from build123d import *

# Parameters (mm, degrees)
SKETCH1_R           = 3.7
BOSS_EXTRUDE1_DEPTH = 3.9
CUT_EXTRUDE1_DEPTH  = 10.392550239
CHAMFER1_SIZE       = 0.4


with BuildPart() as part:
    # Sketch1 → Boss-Extrude1 (new, symmetric)
    with BuildSketch(Plane(origin=(0, 0, 0), x_dir=(1, 0, 0), z_dir=(0, 1, 0))):
        with Locations(Location((0, 0, 0), (0, 0, 270))):
            Circle(SKETCH1_R)
    extrude(amount=BOSS_EXTRUDE1_DEPTH, both=True)

    # Sketch2 → Cut-Extrude1 (cut, through all)
    with BuildSketch(Plane(origin=(0, 3.9, 0), x_dir=(1, 0, 0), z_dir=(0, 1, 0))):
        Polygon((0.925, 0.925), (2.4, 0.925), (2.4, -0.925), (0.925, -0.925), (0.925, -2.4), (-0.925, -2.4), (-0.925, -0.925), (-2.4, -0.925), (-2.4, 0.925), (-0.925, 0.925), (-0.925, 2.4), (0.925, 2.4), align=None)
    extrude(amount=-CUT_EXTRUDE1_DEPTH, mode=Mode.SUBTRACT)

    # Chamfer1
    chamfer1_edges = [part.edges().sort_by_distance(p)[0] for p in [
        (0, -3.9, -3.7),
        (0, 3.9, -3.7),
    ]]
    chamfer(chamfer1_edges, length=CHAMFER1_SIZE)


solid = part.part
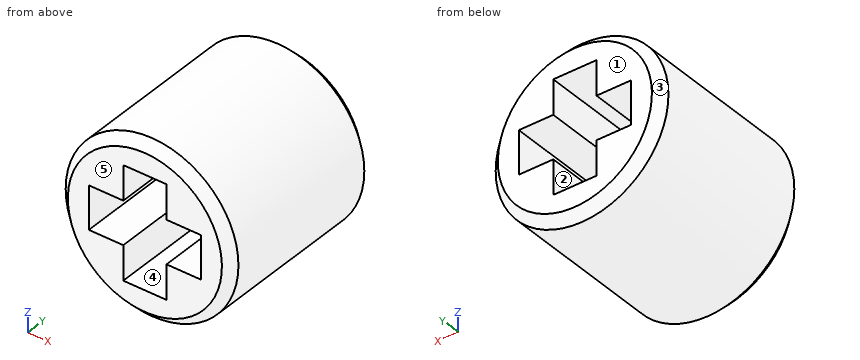
Geometry: final body of the model. Coordinates: model frame, mm. Face numbers are marked on the shaded views. A direction names the side the tool comes from. Give positions to 0.01 mm unless a question says otherwise; leave off trailing zeros. Loops run counter-clockwise (first coordinate to the right, second up) from the corner with the lowest first, then second, coordinate; pieces in that order, holes last. Notation, with made-up numbers: (6, -4.75) -> (20, -4.75) arc R14 cw to (20, 21.25) -> close; hole circle Ø6 at (-18, -17). An arc over 180 degrees is marked (long way). Put each result on its own line as item: value.
1. Cut plane B-B (x = 0). Return the cut outline in (y, z), plus the area to 3 significant figures.
Taken from the geometry:
outline: (-3.9, -3.3) -> (-3.5, -3.7) -> (3.5, -3.7) -> (3.9, -3.3) -> (3.9, -2.4) -> (-3.9, -2.4) -> close; (-3.9, 2.4) -> (3.9, 2.4) -> (3.9, 3.3) -> (3.5, 3.7) -> (-3.5, 3.7) -> (-3.9, 3.3) -> close
area: 20.0 mm2
2. Ray query, line 1 along X through (y, z) = (-0.5, 0); line 2 along X through (y, z) = (-1.25, 1.75) (3 decimals); line 3 along Z through (x, y) = (-1.25, 0.5) (3 decimals). Return the intervals inside material, ascending. Write a range as [from, to].
Taken from the geometry:
line 1: x = [-3.7, -2.4], [2.4, 3.7]
line 2: x = [-3.26, -0.925], [0.925, 3.26]
line 3: z = [-3.482, -0.925], [0.925, 3.482]
3. Pull-direction query (X, two-part tool) for the marked faces 1, 2 and 3; classes: released by +X, released by -X, zero draft, split by the parting line, or undercut.
Taken from the geometry:
face 1: zero draft
face 2: undercut
face 3: split by the parting line
4. Cut plane C-C (y = 0.75). Return the cut outline in (x, z) (3 decimals).
Taken from the geometry:
outline: circle Ø7.4 at (0, 0); hole (-2.4, -0.925) -> (-0.925, -0.925) -> (-0.925, -2.4) -> (0.925, -2.4) -> (0.925, -0.925) -> (2.4, -0.925) -> (2.4, 0.925) -> (0.925, 0.925) -> (0.925, 2.4) -> (-0.925, 2.4) -> (-0.925, 0.925) -> (-2.4, 0.925) -> close
5. Cut plane A-A (z = 0). Return the cut outline in (x, y), plus the area to 3 significant figures.
Taken from the geometry:
outline: (-3.7, -3.5) -> (-3.3, -3.9) -> (-2.4, -3.9) -> (-2.4, 3.9) -> (-3.3, 3.9) -> (-3.7, 3.5) -> close; (2.4, -3.9) -> (3.3, -3.9) -> (3.7, -3.5) -> (3.7, 3.5) -> (3.3, 3.9) -> (2.4, 3.9) -> close
area: 20.0 mm2
6. Pin query (flat end, axial travel): P1, Ø1.6, axis at x = 1.5, y = 0.5, coming from the +Z side; P2, Ø1.2, axis at y = -0.5, z = -2, coming from the -X side; P3, Ø1.2, axis at x = -1.5, y = 0.5, coming from the -Z side; P4, Ø0.9, axis at y = -0.5, z = -0.5, coming from the +X side. Return the tip coordinate at first contact, or that it passes through.
Taken from the geometry:
P1: stops at z = 3.63
P2: stops at x = -3.42
P3: stops at z = -3.59
P4: stops at x = 3.7
7. Set-up query: the marked faces 4 and 5. Return all of +Z, -Z, +X, -X, +Y, -Y with unobstructed straight access to the full face (end or side cutting, diameter ignored); none if empty.
Taken from the geometry:
face 4: +Y, -Y
face 5: +Z, -Z, +X, -X, -Y
